```python
from build123d import *

# Parameters (mm, degrees)
SKETCH_8_W      = 160
SKETCH_8_H      = 40
SKETCH_8_W_2    = 25
SKETCH_8_H_2    = 30
SKETCH_8_W_3    = 90
EXTRUDE_5_DEPTH = 30


with BuildPart() as part:
    # 草图8 → 凸台-拉伸5 (new body)
    with BuildSketch(Plane.XY):
        Rectangle(SKETCH_8_W, SKETCH_8_H)
        with Locations((-62.5, 0)):
            Rectangle(SKETCH_8_W_2, SKETCH_8_H_2, mode=Mode.SUBTRACT)
        with Locations((62.5, 0)):
            Rectangle(SKETCH_8_W_2, SKETCH_8_H_2, mode=Mode.SUBTRACT)
        Rectangle(SKETCH_8_W_3, SKETCH_8_H_2, mode=Mode.SUBTRACT)
    extrude(amount=EXTRUDE_5_DEPTH)


solid = part.part
```
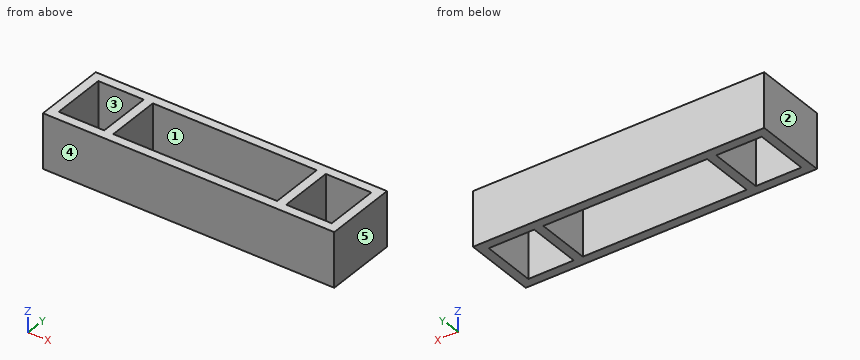
The model under review builds one solid part; all positions refer to its coordinate system, in mm. Face numbers are marked on the shaded views. A direction names the side the tool comes from. Round coordinates to 2 decimals unless told otherwise and drop trailing zeros. Write each loop counter-clockwise with the first axis right and the second up, starting at its lowest first coordinate (ties: lowest second). Pieces come first, ordered by that corner, then holes.
(1) We need section C-C on z = 10.75. Give the boundary of the cut face in (x, y), and give its area (3 significant figures).
(2) Mouldability with a two-part tool opening along Y and no side actions: class the marked faces 3, 4 and 5 as +Y half, -Y half, draft (parallel to the pull), parting line (faces both ways), or undercut.
(3) We need section B-B on x = -18. Give the boundary of the cut face in (y, z), and give its area (3 significant figures).
(4) We need section A-A on y = -5.5. Give the boundary of the cut face in (x, z), and give its area (3 significant figures).
(5) Wall thickness on L1, parallel to X at y = 1.5, z = 2.5; L2, parallel to Y at x = -34, z = 17: over which ranges is each line inside the solid? List them lowest first.
(6) Machinability: for the marked faces 1 and 2, which of the approach directions +Z, -Z, +X, -X, +Y, -Y give a long, thin tool a straight path to every point of the face, cutting with its end or side? Answer none if there is none.
Findings below:
1. outline: (-80, -20) - (80, -20) - (80, 20) - (-80, 20) - close; hole (-75, -15) - (-50, -15) - (-50, 15) - (-75, 15) - close; hole (-45, -15) - (45, -15) - (45, 15) - (-45, 15) - close; hole (50, -15) - (75, -15) - (75, 15) - (50, 15) - close
1. area: 2,200 mm2
2. face 3: undercut
2. face 4: -Y half
2. face 5: draft
3. outline: (-20, 0) - (-15, 0) - (-15, 30) - (-20, 30) - close; (15, 0) - (20, 0) - (20, 30) - (15, 30) - close
3. area: 300 mm2
4. outline: (-80, 0) - (-75, 0) - (-75, 30) - (-80, 30) - close; (-50, 0) - (-45, 0) - (-45, 30) - (-50, 30) - close; (45, 0) - (50, 0) - (50, 30) - (45, 30) - close; (75, 0) - (80, 0) - (80, 30) - (75, 30) - close
4. area: 600 mm2
5. L1: x = -80 to -75, -50 to -45, 45 to 50, 75 to 80
5. L2: y = -20 to -15, 15 to 20
6. face 1: +Z, -Z
6. face 2: +Z, -Z, -X, +Y, -Y
